from build123d import *

# Parameters (mm, degrees)
SKETCH1_W           = 70
SKETCH1_H           = 40
BOSS_EXTRUDE1_DEPTH = 3
CUT_EXTRUDE1_DEPTH  = 3


with BuildPart() as part:
    # Sketch1 → Boss-Extrude1 (new body)
    with BuildSketch(Plane.XY):
        with Locations((35, -20)):
            Rectangle(SKETCH1_W, SKETCH1_H)
    extrude(amount=BOSS_EXTRUDE1_DEPTH)

    # Sketch2 → Cut-Extrude1 (cut)
    with BuildSketch(Plane.XY.offset(3)):
        with BuildLine():
            Line((10, -13), (60, -13))
            ThreePointArc((60, -13), (62, -15), (60, -17))
            Line((60, -17), (10, -17))
            ThreePointArc((10, -17), (8, -15), (10, -13))
        make_face()
    extrude(amount=-CUT_EXTRUDE1_DEPTH, mode=Mode.SUBTRACT)


solid = part.part
For this review, take the finished solid that the model builds, in its own axes (mm). A direction names the side the tool comes from. Give positions to 0.01 mm unless a question says otherwise; leave off trailing zeros. Order: outer loops, then holes, each group sorted by start corner. A loop starts at its lowest first (then second) coordinate and runs counter-clockwise, first axis right, second up. Notation, with made-up numbers: (-2.5, 32) -> (34.5, 32) arc R18 ccw to (34.5, 40) -> close; hole circle Ø11 at (66.25, 81). An arc over 180 degrees is marked (long way). Write item = value, one per line.
1) We need section C-C, the plane z = 0.45. Give the boundary of the cut face in (x, y), and give its area (3 significant figures).
Findings:
outline = (0, -40) -> (70, -40) -> (70, 0) -> (0, 0) -> close; hole (10, -17) -> (60, -17) arc R2 ccw to (60, -13) -> (10, -13) arc R2 ccw to start
area = 2,590 mm^2
2) We need section A-A, the plane x = 15. Give the boundary of the cut face in (y, z).
Findings:
outline = (-40, 0) -> (-17, 0) -> (-17, 3) -> (-40, 3) -> close; (-13, 0) -> (0, 0) -> (0, 3) -> (-13, 3) -> close
3) For faces 5 (the face through (35, -20, 0)), 6 (the face through (62, -15, 2)), list the 3-axis set-ups (+Z, -Z, +X, -X, +Y, -Y) from which the entire face can be reached by the end or side of a thin tool; tool diameter is ignored.
Findings:
face_5 = -Z, +X, -X, +Y, -Y
face_6 = +Z, -Z
4) Insertion check: pin 1 (1 mm diameter, centred on x = 26, y = -14, fed in from +Z). The pin has a flat end and moves straight along its axis. Give the tip position at first contact, or say it passes through.
Findings:
pin_1 = through
5) To check wall thickness, follow L1, parallel to Y at x = 44, z = 0.7; L2, parallel to X at y = -16.5, z = 2.85. State the ranges of each line that lie inside material, in increasing order. Write a range as from..to.
Findings:
L1 = -40..-17, -13..0
L2 = 0..8.68, 61.32..70
6) Draft analysis for pull direction X (two halves, no side actions). For faces 1 (the face through (35, -17, 2)), 2 (the face through (8, -15, 2)), 3 (the face through (0, -20, 1)), 4 (the face through (35, 0, 1)), state which applies: pulls with the +X half, pulls with the -X half, needs draft (parallel to the pull), parting line crosses it, or undercut.
Findings:
face_1 = undercut
face_2 = undercut
face_3 = pulls with the -X half
face_4 = needs draft
7) We need section B-B, the plane y = -15. Give the boundary of the cut face in (x, z), and give its area (3 significant figures).
Findings:
outline = (0, 0) -> (8, 0) -> (8, 3) -> (0, 3) -> close; (62, 0) -> (70, 0) -> (70, 3) -> (62, 3) -> close
area = 48.0 mm^2
